The drawing under review shows one solid part. Ordinate dimensions are in mm from its lowest x, y, z. Round coordinates to 2 decimals unless told otherwise and drop trailing zeros. Write each loop counter-clockwise with the first axis right and the second up, starting at its lowest first coordinate (ties: lowest second). Pieces come first, ordered by that corner, then holes. Notation, with made-up numbers: (45.5, 12) -> (77.5, 12) arc R28 ccw to (77.5, 35) -> close; hole circle Ø5 at (32, 14.5). An arc over 180 degrees is marked (long way). Answer in a Markdown table with one row per item.
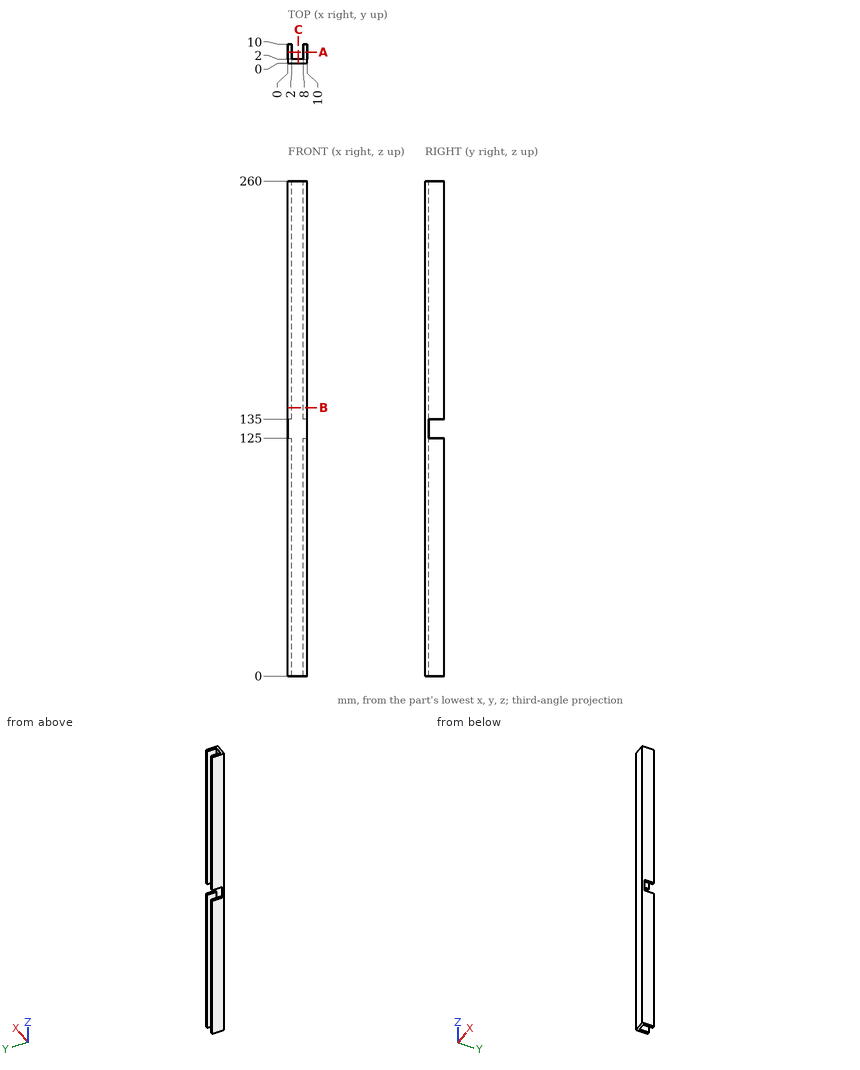
1) Consider section C-C on x = 5.5. State the section outline as (y, z) points.
Solved:
| item | result |
|---|---|
| outline | (0, 0) -> (2, 0) -> (2, 260) -> (0, 260) -> close |
2) Consider section A-A on y = 5.75. State the section outline as (x, z) points.
Solved:
| item | result |
|---|---|
| outline | (0, 0) -> (2, 0) -> (2, 125) -> (0, 125) -> close; (0, 135) -> (2, 135) -> (2, 260) -> (0, 260) -> close; (8, 0) -> (10, 0) -> (10, 125) -> (8, 125) -> close; (8, 135) -> (10, 135) -> (10, 260) -> (8, 260) -> close |
3) Clearance check with a flat-ended pin moving along its axis: pin 1 Ø1 at (x, z) = (7, 142.5) entering from +Y. State where the tip first meets the part, or that it passes through.
Solved:
| item | result |
|---|---|
| pin 1 | y = 2 |
4) Consider section B-B on z = 141. State the section outline as (x, y) points.
Solved:
| item | result |
|---|---|
| outline | (0, 0) -> (10, 0) -> (10, 10) -> (8, 10) -> (8, 2) -> (2, 2) -> (2, 10) -> (0, 10) -> close |
5) For line 1 (X direction, y = 8.75, z = 119); line 2 (Z direction, x = 9, y = 4); line 3 (Y direction, x = 6.25, z = 185.5), list the stretches that pass through material, from the lowest coordinate up. Write a range as [from, to].
Solved:
| item | result |
|---|---|
| line 1 | [0, 2], [8, 10] |
| line 2 | [0, 125], [135, 260] |
| line 3 | [0, 2] |
